Part model, mm, in its own coordinate system. A direction names the side the tool comes from. Give positions to 0.01 mm unless a question says otherwise; leave off trailing zeros. Order: outer loops, then holes, each group sorted by start corner. A loop starts at its lowest first (then second) coordinate and runs counter-clockwise, first axis right, second up. Notation, with made-up numbers: (74.5, 65.5) -> (118.5, 65.5) arc R32 cw to (118.5, 95.5) -> close; hole circle Ø3 at (64.5, -0.5). An arc over 180 degrees is marked (long way). Write item = value, one per line. Start each with the question number.
(1) Saw through at D-D, the plane x = 12. List the corners of the cut face in (y, z), then the cut area to 3 significant figures.
(2) Saw through at A-A, the plane y = 11.5. List the corners of the cut face in (x, z).
(3) Flat gauge pins, fed straight in: pin 1 (5.5 mm diameter, centred on y = 0, z = 37, fed in from -X); pin 2 (4 mm diameter, centred on y = 52, z = -37, fed in from -X); pin 3 (8 mm diameter, centred on x = 12.5, y = 31.5, fed in from +Z); pin 4 (8 mm diameter, centred on x = 8, y = 27, fed in from +Z). Where does each tip first touch, or does it go through?
(4) Saw through at B-B, the plane z = 8.5. List the corners of the cut face in (x, y), then the cut area to 3 significant figures.
(5) Saw through at C-C, the plane x = 47.5. List the corners of the cut face in (y, z).
(6) Which spindle directions (+Z, -Z, +X, -X, +Y, -Y) get a long thin tool onto all of the face, cutting with end or side? Do faces 4 (the cylindrical face through (27.748, 26.467, -11.205)), 5 (the cylindrical face through (27.748, 45.896, -24.448)), 6 (the cylindrical face through (48.76, 0.189, 41.296)), 7 (the flat face through (19.5, 0, 41)). Say none if no direction does.
(7) Probe line 1 along Y through (x, z) = (14, 37); line 2 along Y through (x, z) = (47.75, 37); line 3 along Z through (x, y) = (13, 0). List the from-to ranges inside material, lowest first. Write a range as from..to.
(8) Two-plate mould, pull along X, no slides. Class faces 1 (the flat face through (53, 15, -3)), 2 (the flat face through (46, 5, 2)), 3 (the cylindrical face through (4.93, 1.1, -3.48)): pulls with the +X half, pulls with the -X half, needs draft (parallel to the pull), parting line crosses it, or undercut.
from build123d import *
from build123d.topology import SkipClean

# Parameters (mm, degrees)
SKETCH19_R           = 2.4
SKETCH19_R_2         = 3.65
BASE_DEPTH           = 10
CONNECTOR_DEPTH      = 36
SKETCH21_R           = 2.4
SKETCH21_R_2         = 1.35
THINPLATE_DEPTH      = 7
SPACER_START         = 6
SKETCH22_R           = 3
SKETCH22_R_2         = 1.35
SPACER_DEPTH         = 6
SHOCKHOLE_DEPTH      = 87.821656285
SKETCH25_R           = 2.4
SHOCKSCREWHOLE_DEPTH = 92.836811791
SKETCH26_R           = 4.3
BOLTMOUNT_DEPTH      = 8.6
NUTMOUNT_DEPTH       = 8


with BuildPart() as part:
    # Sketch19 → Base (new body)
    with BuildSketch(Plane(origin=(0, 0, 0), x_dir=(0, 0, -1), z_dir=(1, 0, 0))):
        with BuildLine():
            Line((-37, -8), (0, -10))
            ThreePointArc((0, -10), (4.583911967, -8.887505335), (8.147908412, -5.797550216))
            Line((8.147908412, -5.797550216), (43.51832673, 47.361959827))
            ThreePointArc((43.51832673, 47.361959827), (41.624994171, 58.527589824), (30.463173191, 56.611929669))
            Line((30.463173191, 56.611929669), (7.879284036, 22.669767278))
            Line((7.879284036, 22.669767278), (-22.627449378, 8))
            Line((-22.627449378, 8), (-37, 8))
            ThreePointArc((-37, 8), (-45, 0), (-37, -8))
        make_face()
        with Locations((37, 52)):
            Circle(SKETCH19_R, mode=Mode.SUBTRACT)
        Circle(SKETCH19_R_2, mode=Mode.SUBTRACT)
        with Locations((-37, 0)):
            Circle(SKETCH19_R, mode=Mode.SUBTRACT)
    extrude(amount=BASE_DEPTH)

    # Sketch20 → Connector (add)
    with BuildSketch(Plane(origin=(10, 0, 0), x_dir=(0, 0, -1), z_dir=(1, 0, 0))):
        with BuildLine():
            Line((22.739953466, 45.004417061), (11.476605987, 28.076315503))
            ThreePointArc((11.476605987, 28.076315503), (11.211590252, 26.444347724), (12.265593287, 25.170522865))
            ThreePointArc((12.265593287, 25.170522865), (17.059780993, 22.202789746), (21.162184229, 18.334720032))
            ThreePointArc((21.162184229, 18.334720032), (22.800516777, 17.648363193), (24.338869924, 18.536444744))
            Line((24.338869924, 18.536444744), (36.054780209, 36.144719684))
            ThreePointArc((36.054780209, 36.144719684), (36.228471119, 38.039284164), (34.738265288, 39.22200547))
            ThreePointArc((34.738265288, 39.22200547), (29.8112457, 41.196556117), (26.087002565, 44.97866999))
            ThreePointArc((26.087002565, 44.97866999), (24.420439055, 45.896459743), (22.739953466, 45.004417061))
        make_face()
        with BuildLine():
            Line((-28.142494559, 8), (-37, 8))
            ThreePointArc((-37, 8), (-45, 0), (-37, -8))
            Line((-37, -8), (-28.071624283, -8.482614904))
            ThreePointArc((-28.071624283, -8.482614904), (-27.241263688, -8.114331156), (-27.051523196, -7.22600116))
            ThreePointArc((-27.051523196, -7.22600116), (-27.998959916, -0.241337171), (-27.172063712, 6.75862069))
            ThreePointArc((-27.172063712, 6.75862069), (-27.354655962, 7.615881762), (-28.142494559, 8))
        make_face()
    extrude(amount=CONNECTOR_DEPTH)

    # Sketch21 → ThinPlate (add)
    with BuildSketch(Plane(origin=(46, 0, 0), x_dir=(0, 0, -1), z_dir=(1, 0, 0))):
        with BuildLine():
            Line((-22.627449378, 8), (-28.142494559, 8))
            Line((-28.142494559, 8), (-37, 8))
            ThreePointArc((-37, 8), (-45, 0), (-37, -8))
            Line((-37, -8), (-28.071624283, -8.482614904))
            Line((-28.071624283, -8.482614904), (0, -10))
            ThreePointArc((0, -10), (4.583911967, -8.887505335), (8.147908412, -5.797550216))
            Line((8.147908412, -5.797550216), (24.338869924, 18.536444744))
            Line((24.338869924, 18.536444744), (36.054780209, 36.144719684))
            Line((36.054780209, 36.144719684), (43.51832673, 47.361959827))
            ThreePointArc((43.51832673, 47.361959827), (41.624994171, 58.527589824), (30.463173191, 56.611929669))
            Line((30.463173191, 56.611929669), (22.739953466, 45.004417061))
            Line((22.739953466, 45.004417061), (11.476605987, 28.076315503))
            Line((11.476605987, 28.076315503), (7.879284036, 22.669767278))
            Line((7.879284036, 22.669767278), (-22.627449378, 8))
        make_face()
        with Locations((37, 52)):
            Circle(SKETCH21_R, mode=Mode.SUBTRACT)
        with Locations((-37, 0)):
            Circle(SKETCH21_R, mode=Mode.SUBTRACT)
        Circle(SKETCH21_R_2, mode=Mode.SUBTRACT)
    extrude(amount=THINPLATE_DEPTH)

    # Sketch22 → Spacer (add)
    with SkipClean():  # the faces are left unmerged after this step: merging them gives an invalid solid
        with BuildSketch(Plane.ZY.offset(-46).offset(SPACER_START)):
            with Locations(Location((0, 0, 0), (0, 0, 180))):
                Circle(SKETCH22_R)
            Circle(SKETCH22_R_2, mode=Mode.SUBTRACT)
        extrude(amount=-SPACER_DEPTH)

    # Sketch23 → ShockHole (cut, through all)
    with SkipClean():  # the faces are left unmerged after this step: merging them gives an invalid solid
        with BuildSketch(Plane(origin=(0, 8, 0), x_dir=(1, 0, 0), z_dir=(0, 1, 0))):
            with BuildLine():
                Line((19.5, -37), (19.5, -45.5))
                Line((19.5, -45.5), (36.5, -45.5))
                Line((36.5, -45.5), (36.5, -37))
                ThreePointArc((36.5, -37), (28, -28.5), (19.5, -37))
            make_face()
        extrude(amount=-SHOCKHOLE_DEPTH, mode=Mode.SUBTRACT)

    # Sketch25 → ShockScrewHole (cut, through all)
    with BuildSketch(Plane.ZY):
        with Locations(Location((37, 0, 0), (0, 0, 90))):
            Circle(SKETCH25_R)
    extrude(amount=-SHOCKSCREWHOLE_DEPTH, mode=Mode.SUBTRACT)

    # Sketch26 → BoltMount (cut)
    with SkipClean():  # the faces are left unmerged after this step: merging them gives an invalid solid
        with BuildSketch(Plane(origin=(53, 0, 0), x_dir=(0, 0, -1), z_dir=(1, 0, 0))):
            with Locations((-37, 0)):
                Circle(SKETCH26_R)
        extrude(amount=-BOLTMOUNT_DEPTH, mode=Mode.SUBTRACT)

    # Sketch27 → NutMount (cut)
    with SkipClean():  # the faces are left unmerged after this step: merging them gives an invalid solid
        with BuildSketch(Plane.ZY):
            Polygon((37, -4.387862046), (40.8, -2.193931023), (40.8, 2.193931023), (37, 4.387862046), (33.2, 2.193931023), (33.2, -2.193931023), align=None)
        extrude(amount=-NUTMOUNT_DEPTH, mode=Mode.SUBTRACT)


solid = part.part
Results list:
q1.outline = (-8.48, 28.07) arc R1 ccw to (-7.23, 27.05) arc R28 cw to (6.76, 27.17) arc R1 ccw to (8, 28.14) -> (8, 37) arc R8 ccw to (-8, 37) -> close; (18.33, -21.16) arc R2 ccw to (18.54, -24.34) -> (36.14, -36.05) arc R2 ccw to (39.22, -34.74) arc R12.98 cw to (44.98, -26.09) arc R2 ccw to (45, -22.74) -> (28.08, -11.48) arc R2 ccw to (25.17, -12.27) arc R28 cw to start; hole circle Ø4.8 at (0, 37)
q1.area = 613 mm^2
q2.outline = (0, -19.66) -> (10, -19.66) -> (10, 15.35) -> (0, 15.35) -> close; (46, -19.66) -> (53, -19.66) -> (53, 15.35) -> (46, 15.35) -> close
q3.pin_1 = 8
q3.pin_2 = through
q3.pin_3 = -11.21
q3.pin_4 = -8.1
q4.outline = (0, -9.54) -> (10, -9.54) -> (10, 14.79) -> (0, 14.79) -> close; (46, -9.54) -> (53, -9.54) -> (53, 14.79) -> (46, 14.79) -> close
q4.area = 414 mm^2
q5.outline = (-10, 0) arc R10 ccw to (-5.8, -8.15) -> (47.36, -43.52) arc R8 ccw to (56.61, -30.46) -> (22.67, -7.88) -> (8, 22.63) -> (8, 37) arc R8 ccw to (-8, 37) -> close; hole circle Ø8.6 at (0, 37); hole circle Ø2.7 at (0, 0); hole circle Ø4.8 at (52, -37)
q6.face_4 = +Z
q6.face_5 = +Y
q6.face_6 = +X
q6.face_7 = +Z, +Y, -Y
q7.line_1 = -8..-2.4, 2.4..8
q7.line_2 = -8..-4.3, 4.3..8
q7.line_3 = 28..34.6, 39.4..45
q8.face_1 = pulls with the +X half
q8.face_2 = undercut
q8.face_3 = needs draft
